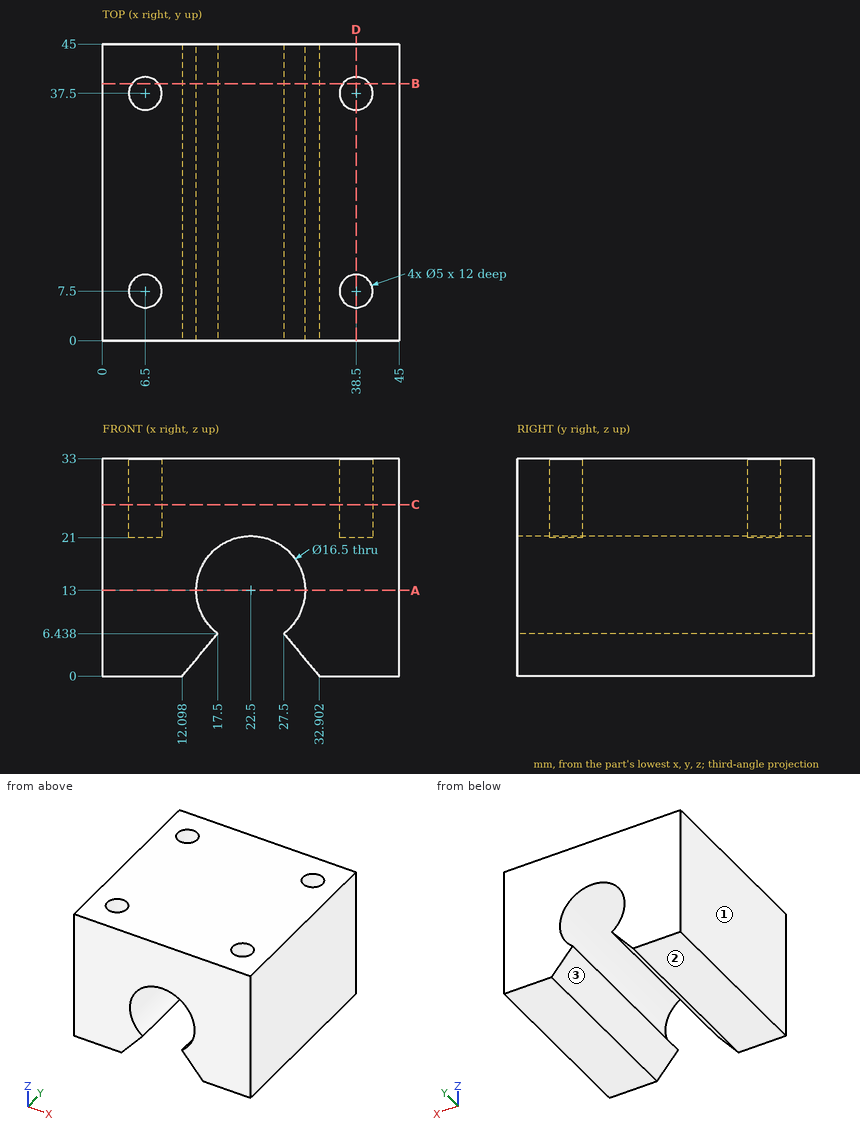
Source: three-view drawing plus pictorial views. Frame: mm from the lowest corner of the part. Coordinates: 2 decimals unless noted, no trailing zeros. Loops run counter-clockwise (first coordinate to the right, second up) from the corner with the lowest first, then second, coordinate; pieces in that order, holes last. Notation, with made-up numbers: (25.5, 77) - (30.5, 77) arc R25 ccw to (30.5, 107) - close; hole circle Ø1 at (35.5, 37). An arc over 180 degrees is marked (long way). One line per item, written item: value. Start each with the question number.
1. Section C-C (z = 26). Return the cut outline in (x, y), and give its area (3 significant figures).
2. Ray query, L1, parallel to Y at x = 38.5, z = 26.25; L2, parallel to Y at x = 38, z = 25; L3, parallel to X at y = 37, z = 30. Return the intervals inside material, ascending.
3. Section B-B (y = 39). Return the cut outline in (x, z).
4. Mould query, pull axis X, two halves, no side actions, for the marked faces 1, 2 and 3. Classes: pulls with the +X half, pulls with the -X half, needs draft (parallel to the pull), parting line crosses it, or undercut.
5. Section A-A (z = 13). Return the cut outline in (x, y).
6. Section D-D (x = 38.5). Return the cut outline in (y, z), and give its area (4 significant figures).
7. Contact query for a flat-ended pin moving along its axis: P1, Ø1.5, axis at x = 7, y = 38.5, coming from the +Z side. Output: stop coordinate, or through.
Verdict:
1. outline: (0, 0) - (45, 0) - (45, 45) - (0, 45) - close; hole circle Ø5 at (6.5, 7.5); hole circle Ø5 at (6.5, 37.5); hole circle Ø5 at (38.5, 7.5); hole circle Ø5 at (38.5, 37.5)
1. area: 1,950 mm2
2. L1: y = 0 to 5, 10 to 35, 40 to 45
2. L2: y = 0 to 5.05, 9.95 to 35.05, 39.95 to 45
2. L3: x = 0 to 4.05, 8.95 to 36.05, 40.95 to 45
3. outline: (0, 0) - (12.1, 0) - (17.5, 6.44) arc R8.25 cw (long way) to (27.5, 6.44) - (32.9, 0) - (45, 0) - (45, 33) - (40.5, 33) - (40.5, 21) - (36.5, 21) - (36.5, 33) - (8.5, 33) - (8.5, 21) - (4.5, 21) - (4.5, 33) - (0, 33) - close
4. face 1: pulls with the -X half
4. face 2: needs draft
4. face 3: undercut
5. outline: (0, 0) - (14.25, 0) - (14.25, 45) - (0, 45) - close; (30.75, 0) - (45, 0) - (45, 45) - (30.75, 45) - close
6. outline: (0, 0) - (45, 0) - (45, 33) - (40, 33) - (40, 21) - (35, 21) - (35, 33) - (10, 33) - (10, 21) - (5, 21) - (5, 33) - (0, 33) - close
6. area: 1,365 mm2
7. P1: stops at z = 21
